Here's how the part is built. I have some questions about the finished solid (model axes, mm). Face numbers are marked on the shaded views. A direction names the side the tool comes from. Coordinates: 2 decimals unless noted, no trailing zeros. Loops run counter-clockwise (first coordinate to the right, second up) from the corner with the lowest first, then second, coordinate; pieces in that order, holes last. Notation, with made-up numbers: M 43,25 L 86,25 A24 ccw 86,44 Z; hole C 53.5,83.5 d8. An arc over 180 degrees is marked long. Use one line per item in the form item = value. Start each with the question number.
(1) Imagine slicing it at A-A, the plane y = -6.5. Please give me the cut outline in (x, z), and give its area (3 significant figures).
(2) Will these pins go through, and if not, where does the flat tip stop? P1, Ø4, axis at y = 4.5, z = 3.5, coming from the +X side; P2, Ø2, axis at y = 2.5, z = 4, coming from the -X side; P3, Ø0.6, axis at x = 31.5, y = -8, coming from the +Z side; P4, Ø1.2, axis at x = 17, z = 3, coming from the +Y side.
(3) On a 3-axis mill with a long thin cutter (end or side, diameter ignored), from which of +Z, -Z, +X, -X, +Y, -Y can I reach the whole of each face in a straight line? I mean the marked faces 5 and 6. Say none if no direction works.
(4) Imagine slicing it at B-B, the plane x = -15. Please give me the cut outline in (y, z).
(5) Please list where these lines run through material, in increasing order: L1, parallel to X at y = -4.5, z = 1; L2, parallel to Y at x = -11.5, z = 2.25; L3, parallel to X at y = 3.5, z = 4.
(6) Thinking about a two-plate mould opening in X: for the marked faces 1, 2, 3 and 4, which applies, +X half, -X half, draft (parallel to the pull), parting line (faces both ways), or undercut?
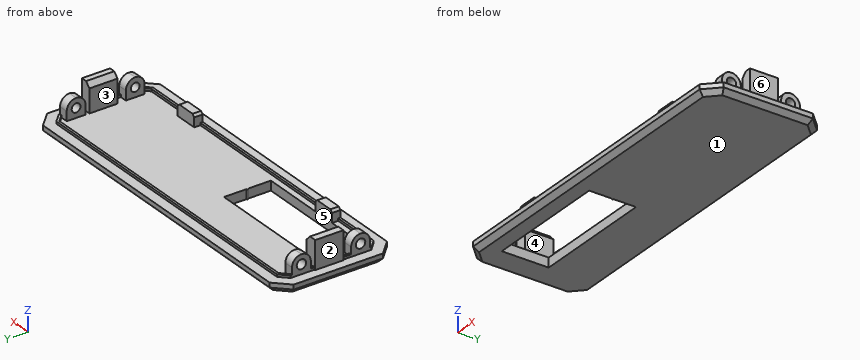
```python
from build123d import *

# Parameters (mm, degrees)
EXTRUDE_1_DEPTH               = 2
CHAMFER_1_SIZE                = 1
SKETCH_3_W                    = 2
SKETCH_3_H                    = 4
EXTRUDE_2_DEPTH               = 4
FILLET_1_R                    = 2
SKETCH_4_R                    = 1
CUT_EXTRUDE_1_DEPTH           = 2
CUT_EXTRUDE_1_DRAFT           = -2
CUT_EXTRUDE_1_PROFILE_2_DEPTH = 2
CUT_EXTRUDE_1_PROFILE_2_DRAFT = -2
SKETCH_5_R                    = 1
CUT_EXTRUDE_2_DEPTH           = 2
CUT_EXTRUDE_2_DRAFT           = -2
CUT_EXTRUDE_2_PROFILE_2_DEPTH = 2
CUT_EXTRUDE_2_PROFILE_2_DRAFT = -2
SKETCH_8_W                    = 2.55
SKETCH_8_H                    = 6
SKETCH_8_W_2                  = 2.25
EXTRUDE_5_DEPTH               = 6
CHAMFER_3_SIZE                = 1
CUT_EXTRUDE_3_REACH           = 46.057
SKETCH_10_W                   = 26.2
SKETCH_10_H                   = 10
EXTRUDE_7_DEPTH               = 0.5
SKETCH_12_W                   = 4.95
SKETCH_12_H                   = 1.8
EXTRUDE_8_DEPTH               = 2.5
CHAMFER_4_SIZE                = 0.5
SKETCH_13_R                   = 0.2
EXTRUDE_9_DEPTH               = 2


with BuildPart() as part:
    # 草图1 → 凸台-拉伸1 (new body)
    with BuildSketch(Plane.XY):
        Polygon((-39.76383505, 4.799206062), (-36.76383505, 7.799206062), (31.23616495, 7.799206062), (34.23616495, 4.799206062), (34.23616495, -14.200793938), (31.23616495, -17.200793938), (-36.76383505, -17.200793938), (-39.76383505, -14.200793938), align=None)
    extrude(amount=EXTRUDE_1_DEPTH)

    # 倒角1
    chamfer_1_edges = [part.edges().sort_by_distance(p)[0] for p in [
        (-38.26383505, -15.700793938, 0),
        (-39.76383505, -4.700793938, 0),
        (-38.26383505, 6.299206062, 0),
        (-2.76383505, 7.799206062, 0),
        (32.73616495, 6.299206062, 0),
        (34.23616495, -4.700793938, 0),
        (32.73616495, -15.700793938, 0),
        (-2.76383505, -17.200793938, 0),
    ]]
    chamfer(chamfer_1_edges, length=CHAMFER_1_SIZE)

    # 草图3 → 凸台-拉伸2 (add)
    with BuildSketch(Plane.XY.offset(2)):
        with Locations((-36.56383505, 1.599206062)):
            Rectangle(SKETCH_3_W, SKETCH_3_H)
        with Locations((-36.56383505, -11.000793938)):
            Rectangle(SKETCH_3_W, SKETCH_3_H)
        with Locations((31.03616495, 1.599206062)):
            Rectangle(SKETCH_3_W, SKETCH_3_H)
        with Locations((31.03616495, -11.000793938)):
            Rectangle(SKETCH_3_W, SKETCH_3_H)
    extrude(amount=EXTRUDE_2_DEPTH)

    # 圆角1
    fillet_1_edges = [part.edges().sort_by_distance(p)[0] for p in [
        (31.03616495, 3.599206062, 6),
        (31.03616495, -0.400793938, 6),
        (31.03616495, -9.000793938, 6),
        (31.03616495, -13.000793938, 6),
        (-36.56383505, -13.000793938, 6),
        (-36.56383505, -9.000793938, 6),
        (-36.56383505, 3.599206062, 6),
        (-36.56383505, -0.400793938, 6),
    ]]
    fillet(fillet_1_edges, radius=FILLET_1_R - 0.0001)  # a hair under: the kernel refuses the full size


with BuildPart() as cut_extrude_1_tool:
    # 草图4 → 切除-拉伸1 (with draft: the straight prism first)
    with BuildSketch(Plane(origin=(32.03616495, 0, 0), x_dir=(0, 0, -1), z_dir=(1, 0, 0))):
        with Locations((-4, 1.599206062)):
            Circle(SKETCH_4_R)
    extrude(amount=-CUT_EXTRUDE_1_DEPTH)
    # 切除-拉伸1: the draft: its side faces are tilted about the plane it starts from
    cut_extrude_1_sides = [cut_extrude_1_tool.faces().sort_by_distance(p)[0] for p in [
        (31.03616495, 1.599206062, 5),
    ]]
    draft(cut_extrude_1_sides, Plane(origin=(32.03616495, 0, 0), x_dir=(0, 0, -1), z_dir=(1, 0, 0)), CUT_EXTRUDE_1_DRAFT)


with BuildPart() as part_1:
    add(part.part)

    # 切除-拉伸1: cut by cut_extrude_1_tool
    add(cut_extrude_1_tool.part, mode=Mode.SUBTRACT)


with BuildPart() as cut_extrude_1_profile_2_tool:
    # 草图4 → 切除-拉伸1 profile 2 (with draft: the straight prism first)
    with BuildSketch(Plane(origin=(32.03616495, 0, 0), x_dir=(0, 0, -1), z_dir=(1, 0, 0))):
        with Locations((-4, -11.000793938)):
            Circle(SKETCH_4_R)
    extrude(amount=-CUT_EXTRUDE_1_PROFILE_2_DEPTH)
    # 切除-拉伸1 profile 2: the draft: its side faces are tilted about the plane it starts from
    cut_extrude_1_profile_2_sides = [cut_extrude_1_profile_2_tool.faces().sort_by_distance(p)[0] for p in [
        (31.03616495, -11.000793938, 5),
    ]]
    draft(cut_extrude_1_profile_2_sides, Plane(origin=(32.03616495, 0, 0), x_dir=(0, 0, -1), z_dir=(1, 0, 0)), CUT_EXTRUDE_1_PROFILE_2_DRAFT)


with BuildPart() as part_2:
    add(part_1.part)

    # 切除-拉伸1 profile 2: cut by cut_extrude_1_profile_2_tool
    add(cut_extrude_1_profile_2_tool.part, mode=Mode.SUBTRACT)


with BuildPart() as cut_extrude_2_tool:
    # 草图5 → 切除-拉伸2 (with draft: the straight prism first)
    with BuildSketch(Plane.ZY.offset(37.56383505)):
        with Locations((4, 1.599206062)):
            Circle(SKETCH_5_R)
    extrude(amount=-CUT_EXTRUDE_2_DEPTH)
    # 切除-拉伸2: the draft: its side faces are tilted about the plane it starts from
    cut_extrude_2_sides = [cut_extrude_2_tool.faces().sort_by_distance(p)[0] for p in [
        (-36.56383505, 1.599206062, 3),
    ]]
    draft(cut_extrude_2_sides, Plane.ZY.offset(37.56383505), CUT_EXTRUDE_2_DRAFT)


with BuildPart() as part_3:
    add(part_2.part)

    # 切除-拉伸2: cut by cut_extrude_2_tool
    add(cut_extrude_2_tool.part, mode=Mode.SUBTRACT)


with BuildPart() as cut_extrude_2_profile_2_tool:
    # 草图5 → 切除-拉伸2 profile 2 (with draft: the straight prism first)
    with BuildSketch(Plane.ZY.offset(37.56383505)):
        with Locations((4, -11.000793938)):
            Circle(SKETCH_5_R)
    extrude(amount=-CUT_EXTRUDE_2_PROFILE_2_DEPTH)
    # 切除-拉伸2 profile 2: the draft: its side faces are tilted about the plane it starts from
    cut_extrude_2_profile_2_sides = [cut_extrude_2_profile_2_tool.faces().sort_by_distance(p)[0] for p in [
        (-36.56383505, -11.000793938, 3),
    ]]
    draft(cut_extrude_2_profile_2_sides, Plane.ZY.offset(37.56383505), CUT_EXTRUDE_2_PROFILE_2_DRAFT)


with BuildPart() as part_4:
    add(part_3.part)

    # 切除-拉伸2 profile 2: cut by cut_extrude_2_profile_2_tool
    add(cut_extrude_2_profile_2_tool.part, mode=Mode.SUBTRACT)

    # 草图8 → 凸台-拉伸5 (add)
    with BuildSketch(Plane.XY.offset(2)):
        with Locations((-36.48883505, -4.200793938)):
            Rectangle(SKETCH_8_W, SKETCH_8_H)
        with Locations((31.11116495, -4.200793938)):
            Rectangle(SKETCH_8_W_2, SKETCH_8_H)
    extrude(amount=EXTRUDE_5_DEPTH)

    # 倒角3
    chamfer_3_edges = [part_4.edges().sort_by_distance(p)[0] for p in [
        (-35.21383505, -4.200793938, 8),
        (29.98616495, -4.200793938, 8),
    ]]
    chamfer(chamfer_3_edges, length=CHAMFER_3_SIZE)

    # 草图10 → 切除-拉伸3 (cut, up to next)
    with BuildSketch(Plane(origin=(0, 0, 0), x_dir=(-1, 0, 0), z_dir=(0, 0, -1)), mode=Mode.PRIVATE) as cut_extrude_3_sk1:
        with Locations((20.66383505, -8.200793938)):
            Rectangle(SKETCH_10_W, SKETCH_10_H)
    cut_extrude_3_tool1 = extrude(cut_extrude_3_sk1.sketch, amount=-CUT_EXTRUDE_3_REACH, mode=Mode.PRIVATE) & part_4.part
    add(cut_extrude_3_tool1.solids().sort_by_distance((-20.663835, -8.200794, 0))[0], mode=Mode.SUBTRACT)

    # 草图11 → 凸台-拉伸7 (add)
    with BuildSketch(Plane.XY.offset(2)):
        Polygon((30.324895113, 5.599206062), (-35.852565213, 5.599206062), (-37.56383505, 3.887936224), (-37.56383505, -13.289524101), (-35.852565213, -15.000793938), (30.324895113, -15.000793938), (32.03616495, -13.289524101), (32.03616495, 3.887936224), align=None)
        Polygon((30.117788331, 5.099206062), (-35.645458432, 5.099206062), (-37.06383505, 3.680829443), (-37.06383505, -13.08241732), (-35.645458432, -14.500793938), (30.117788331, -14.500793938), (31.53616495, -13.08241732), (31.53616495, 3.680829443), align=None, mode=Mode.SUBTRACT)
    extrude(amount=EXTRUDE_7_DEPTH)

    # 草图12 → 凸台-拉伸8 (add)
    with BuildSketch(Plane.XY.offset(2)):
        with Locations((17.91116495, -14.100793938)):
            Rectangle(SKETCH_12_W, SKETCH_12_H)
        with Locations((-23.43883505, -14.100793938)):
            Rectangle(SKETCH_12_W, SKETCH_12_H)
    extrude(amount=EXTRUDE_8_DEPTH)

    # 倒角4
    chamfer_4_edges = [part_4.edges().sort_by_distance(p)[0] for p in [
        (15.43616495, -14.100793938, 4.5),
        (20.38616495, -14.100793938, 4.5),
        (-25.91383505, -14.100793938, 4.5),
        (-20.96383505, -14.100793938, 4.5),
    ]]
    chamfer(chamfer_4_edges, length=CHAMFER_4_SIZE)

    # 草图13 → 凸台-拉伸9 (add)
    with BuildSketch(Plane(origin=(0, 0, 0), x_dir=(-1, 0, 0), z_dir=(0, 0, -1))):
        with Locations((7.56383505, -8.200793938)):
            Circle(SKETCH_13_R)
    extrude(amount=-EXTRUDE_9_DEPTH)


solid = part_4.part
```
Answer:
q1.outline = M -39.76,1 L -38.76,0 L -33.76,0 L -33.76,2 L -35.21,2 L -35.21,7 L -36.21,8 L -37.76,8 L -37.76,2 L -39.76,2 Z; M -7.56,0 L 33.24,0 L 34.24,1 L 34.24,2 L 32.24,2 L 32.24,8 L 30.99,8 L 29.99,7 L 29.99,2 L -7.56,2 Z
q1.area = 122 mm²
q2.P1 = 34.24
q2.P2 = -37.56
q2.P3 = 2.5
q2.P4 = 5.6
q3.face_5 = +Z, -Z
q3.face_6 = +Z, +X, +Y, -Y
q4.outline = M -17.2,1 L -16.2,0 L -13.2,0 L -13.2,2 L -14.5,2 L -14.5,2.5 L -15,2.5 L -15,2 L -17.2,2 Z; M -3.2,0 L 6.8,0 L 7.8,1 L 7.8,2 L 5.6,2 L 5.6,2.5 L 5.1,2.5 L 5.1,2 L -3.2,2 Z
q5.L1 = -39.76 to -33.76, -7.56 to 34.24
q5.L2 = -15 to -14.5, 5.1 to 5.6
q5.L3 = -37.56 to -35.56, 30.04 to 32.04
q6.face_1 = draft
q6.face_2 = -X half
q6.face_3 = undercut
q6.face_4 = undercut
